Here's the drawing with two shaded views (mm, measured from the low corner). I have some questions. A direction names the side the tool comes from. Give positions to 0.01 mm unless a question says otherwise; leave off trailing zeros. Write each loop counter-clockwise with the first axis right and the second up, starting at its lowest first coordinate (ties: lowest second). Pieces come first, ordered by that corner, then holes. Notation, with made-up numbers: M 77.25,15.5 L 92.25,15.5 A23 cw 92.25,42.5 Z; hole C 32,28 d9. An arc over 180 degrees is marked long. Answer as CSV lines item,"result". Start each with the question number.
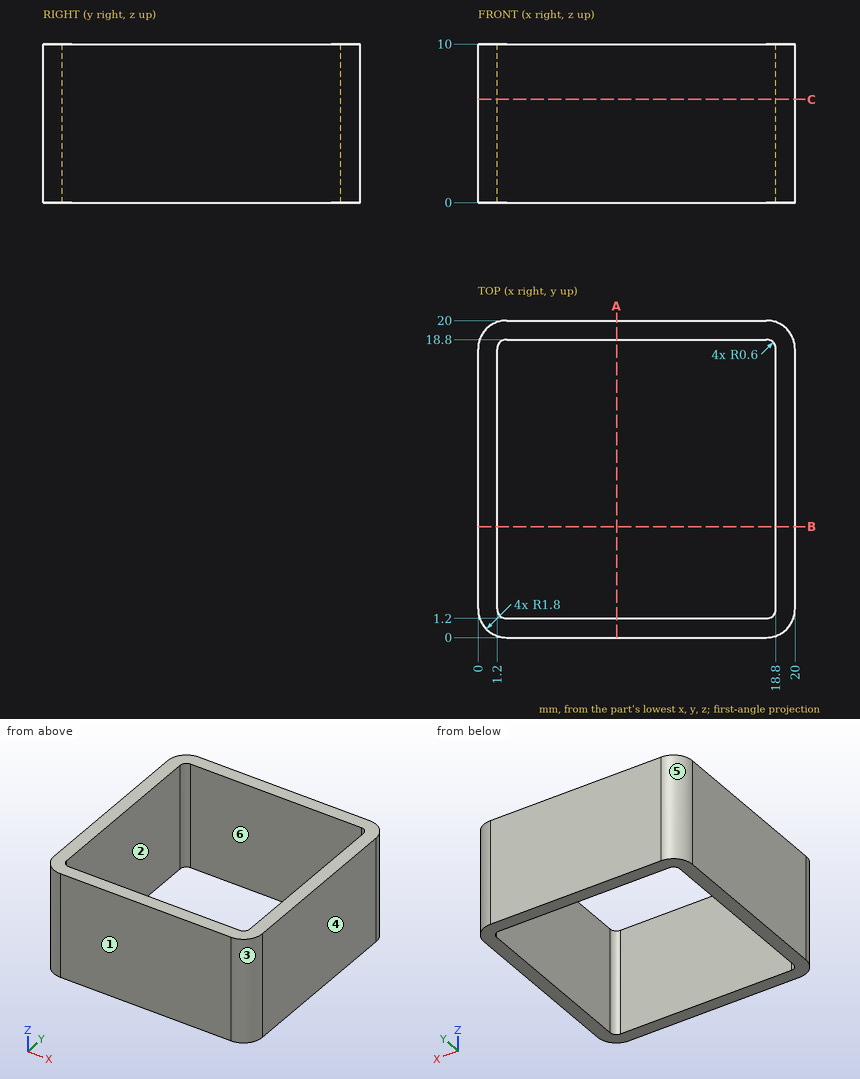
1. Please list where these lines run through material, in increasing order: line 1 (X direction, y = 3.5, z = 7.5); line 2 (X direction, y = 18.5, z = 4.75).
2. Imagine slicing it at A-A, the plane x = 8.75. Please give me the cut outline in (y, z), plus the area to 3 significant figures.
3. On a 3-axis mill with a long thin cutter (end or side, diameter ignored), from which of +Z, -Z, +X, -X, +Y, -Y can I reach the whole of each face in a straight line? I mean the marked faces 1 and 2. Say none if no direction works.
4. Will this pin go through, and if not, where does the flat tip stop? P1, Ø5, axis at x = 16, y = 13.5, coming from the +Z side.
5. Imagine slicing it at C-C, the plane z = 6.5. Please give me the cut outline in (x, y), plus the area to 3 significant figures.
6. Thinking about a two-plate mould opening in Y: for the marked faces 3, 4, 5 and 6, which applies, pulls with the +Y half, pulls with the -Y half, needs draft (parallel to the pull), parting line crosses it, or undercut?
Solutions:
1,line 1,"0 to 1.2, 18.8 to 20"
1,line 2,"0.03 to 1.28, 18.72 to 19.97"
2,outline,"M 0,0 L 1.2,0 L 1.2,10 L 0,10 Z; M 18.8,0 L 20,0 L 20,10 L 18.8,10 Z"
2,area,"24.0 mm²"
3,face 1,"+Z, -Z, +X, -X, -Y"
3,face 2,"+Z, -Z"
4,P1,"through"
5,outline,"M 0,1.8 A1.8 ccw 1.8,0 L 18.2,0 A1.8 ccw 20,1.8 L 20,18.2 A1.8 ccw 18.2,20 L 1.8,20 A1.8 ccw 0,18.2 Z; hole M 1.2,1.8 A0.6 ccw 1.8,1.2 L 18.2,1.2 A0.6 ccw 18.8,1.8 L 18.8,18.2 A0.6 ccw 18.2,18.8 L 1.8,18.8 A0.6 ccw 1.2,18.2 Z"
5,area,"87.8 mm²"
6,face 3,"pulls with the -Y half"
6,face 4,"needs draft"
6,face 5,"pulls with the +Y half"
6,face 6,"undercut"
